from build123d import *

# Parameters (mm, degrees)
SALIENTE_EXTRUIR1_DEPTH = 18
CROQUIS2_R              = 36
SALIENTE_EXTRUIR2_DEPTH = 15
CROQUIS3_R              = 31
CORTAR_EXTRUIR1_DEPTH   = 21
CROQUIS4_R              = 25
CORTAR_EXTRUIR2_DEPTH   = 21
CROQUIS5_R              = 3.25
CORTAR_EXTRUIR3_DEPTH   = 21
MATRIZC1_COUNT          = 6
CROQUIS6_R              = 5
CORTAR_EXTRUIR4_DEPTH   = 6
MATRIZC2_COUNT          = 6
CROQUIS7_R              = 3.25
CORTAR_EXTRUIR5_DEPTH   = 27


with BuildPart() as part:
    # Croquis1 → Saliente-Extruir1 (new body)
    with BuildSketch(Plane.XY):
        with BuildLine():
            Line((-21.794494718, 45), (21.794494718, 45))
            ThreePointArc((21.794494718, 45), (0, -50), (-21.794494718, 45))
        make_face()
    extrude(amount=SALIENTE_EXTRUIR1_DEPTH)

    # Croquis2 → Saliente-Extruir2 (add)
    with BuildSketch(Plane.XY.offset(18)):
        Circle(CROQUIS2_R)
    extrude(amount=SALIENTE_EXTRUIR2_DEPTH)

    # Croquis3 → Cortar-Extruir1 (cut)
    with BuildSketch(Plane(origin=(0, 0, 0), x_dir=(-1, 0, 0), z_dir=(0, 0, -1))):
        Circle(CROQUIS3_R)
    extrude(amount=-CORTAR_EXTRUIR1_DEPTH, mode=Mode.SUBTRACT)

    # Croquis4 → Cortar-Extruir2 (cut)
    with BuildSketch(Plane(origin=(0, 0, 21), x_dir=(-1, 0, 0), z_dir=(0, 0, -1))):
        Circle(CROQUIS4_R)
    extrude(amount=-CORTAR_EXTRUIR2_DEPTH, mode=Mode.SUBTRACT)

    # Croquis5 → Cortar-Extruir3 (cut)
    with BuildSketch(Plane(origin=(0, 0, 0), x_dir=(-1, 0, 0), z_dir=(0, 0, -1))):
        with Locations((-42, 0)):
            Circle(CROQUIS5_R)
    cortar_extruir3 = extrude(amount=-CORTAR_EXTRUIR3_DEPTH, mode=Mode.SUBTRACT)

    # MatrizC1: Cortar-Extruir3 ×6 about axis
    matrizc1_axis = Axis((0, 0, 0), (0, 0, 1))
    for i in range(1, MATRIZC1_COUNT):
        add(cortar_extruir3.rotate(matrizc1_axis, i * 360 / MATRIZC1_COUNT), mode=Mode.SUBTRACT)

    # Croquis6 → Cortar-Extruir4 (cut)
    with BuildSketch(Plane(origin=(0, 0, 0), x_dir=(-1, 0, 0), z_dir=(0, 0, -1))):
        with Locations((-21, 36.373066959)):
            Circle(CROQUIS6_R)
    cortar_extruir4 = extrude(amount=-CORTAR_EXTRUIR4_DEPTH, mode=Mode.SUBTRACT)

    # MatrizC2: Cortar-Extruir4 ×6 about axis
    matrizc2_axis = Axis((0, 0, 0), (0, 0, 1))
    for i in range(1, MATRIZC2_COUNT):
        add(cortar_extruir4.rotate(matrizc2_axis, i * 360 / MATRIZC2_COUNT), mode=Mode.SUBTRACT)

    # Croquis7 → Cortar-Extruir5 (cut)
    with BuildSketch(Plane(origin=(0, 45, 0), x_dir=(1, 0, 0), z_dir=(0, 1, 0))):
        with Locations((0, -24)):
            Circle(CROQUIS7_R)
    extrude(amount=-CORTAR_EXTRUIR5_DEPTH, mode=Mode.SUBTRACT)


solid = part.part
Work out the finished part from the listing and answer in its coordinate system (mm). A direction names the side the tool comes from. Round coordinates to 2 decimals unless told otherwise and drop trailing zeros. Loops run counter-clockwise (first coordinate to the right, second up) from the corner with the lowest first, then second, coordinate; pieces in that order, holes last. Notation, with made-up numbers: (73.25, -5.5) -> (122.25, -5.5) arc R15 cw to (122.25, 20.5) -> close; hole circle Ø7 at (50, 29.5). An arc over 180 degrees is marked (long way). Use one line per item in the form item = value.
(1) For a pull along Y with two mould halves and no side action, classify faces 4 (the flat face through (-25, -7, 33)), 5 (the cylindrical face through (21.65, 41.33, 2.96)), 6 (the flat face through (-18.7, 33.8, 6)) as released by +Y, released by -Y, zero draft, split by the parting line, or undercut.
Answer list:
face_4 = zero draft
face_5 = undercut
face_6 = undercut
(2) Find section A-A on y = 0. Give the number of separate pieces and of enclosed holes in the cut face, then the cut area to 3 significant figures.
Answer list:
separate_pieces = 4
enclosed_holes = 0
area = 702 mm2
(3) Find section C-C on y = -20. Give the vertices of the cut face in (x, z), then the cut area to 3 significant figures.
Answer list:
outline = (-45.83, 0) -> (-23.69, 0) -> (-23.69, 21) -> (-15, 21) -> (-15, 33) -> (-29.93, 33) -> (-29.93, 18) -> (-45.83, 18) -> close; (15, 21) -> (23.69, 21) -> (23.69, 0) -> (45.83, 0) -> (45.83, 18) -> (29.93, 18) -> (29.93, 33) -> (15, 33) -> close
area = 1,190 mm2
(4) Find section B-B on x = 0. Give the vertices of the cut face in (y, z), then the cut area to 3 significant figures.
Answer list:
outline = (-50, 0) -> (-31, 0) -> (-31, 21) -> (-25, 21) -> (-25, 33) -> (-36, 33) -> (-36, 18) -> (-50, 18) -> close; (25, 27.25) -> (36, 27.25) -> (36, 33) -> (25, 33) -> close; (31, 0) -> (45, 0) -> (45, 18) -> (36, 18) -> (36, 20.75) -> (31, 20.75) -> close
area = 818 mm2
(5) A tool of negligible diameter and unlimited length cuts with its end or side. For faces 1 (the cylindrical face through (-23.846, 7.509, 26.916)), 2 (the cylindrical face through (-0.705, 30.474, 27.173)), 3 (the flat face through (-17.7, -35.3, 6)), from which of +Z, -Z, +X, -X, +Y, -Y can it reach the whole face along a straight path? Write none if from no direction.
Answer list:
face_1 = +Z, -Z
face_2 = +Y
face_3 = -Z
(6) Flat-ended cylindrical pins translate along their axes: P1, Ø3, axis at y = -23.5, z = 21.5, coming from the +X side; P2, Ø12, axis at x = 23, z = 28.5, coming from the +Y side; P3, Ø3, axis at x = -43.5, y = -2.5, coming from the -Z side; P4, Ø18.5, axis at x = -13, y = 2, coming from the -Z side. Find the tip coordinate at first contact, or state that the pin passes through.
Answer list:
P1 = 28.5
P2 = 31.73
P3 = 6
P4 = through
(7) Straight lines are drawn through the part: line 1 (Y direction, x = 0, z = 27.5); line 2 (Y direction, x = 21, z = 14.5); line 3 (Z direction, x = -34, y = 20). For each, find the intervals that lie inside material, in ascending order.
Answer list:
line_1 = -36 to -25, 25 to 36
line_2 = -45.38 to -39.62, -33.12 to -22.8, 22.8 to 33.12, 39.62 to 45
line_3 = 0 to 18
